```python
from build123d import *

# Parameters (mm, degrees)
BOSS_EXTRUDE1_DEPTH = 80
FILLET1_R           = 1
SKETCH4_R           = 2.05
BOSS_EXTRUDE2_DEPTH = 3.5
BOSS_EXTRUDE3_START = -15
BOSS_EXTRUDE3_DEPTH = 15
SKETCH6_R           = 3.25
CUT_EXTRUDE1_DEPTH  = 44.5
SKETCH8_R           = 1.65
CUT_EXTRUDE2_DEPTH  = 179.465826414


with BuildPart() as part:
    # Sketch1 → Boss-Extrude1 (new body)
    with BuildSketch(Plane.XY):
        with BuildLine():
            Line((-141.65, 83.343364131), (-141.65, 117.256635869))
            Line((-141.65, 117.256635869), (-141.65, 119.95))
            ThreePointArc((-141.65, 119.95), (-141.064213562, 121.364213562), (-139.65, 121.95))
            Line((-139.65, 121.95), (-136.956635869, 121.95))
            Line((-136.956635869, 121.95), (-103.043364131, 121.95))
            Line((-103.043364131, 121.95), (-100.35, 121.95))
            ThreePointArc((-100.35, 121.95), (-98.935786438, 121.364213562), (-98.35, 119.95))
            Line((-98.35, 119.95), (-98.35, 117.256635869))
            Line((-98.35, 117.256635869), (-98.35, 83.343364131))
            Line((-98.35, 83.343364131), (-98.35, 80.65))
            ThreePointArc((-98.35, 80.65), (-98.935786438, 79.235786438), (-100.35, 78.65))
            Line((-100.35, 78.65), (-103.043364131, 78.65))
            Line((-103.043364131, 78.65), (-107.615836726, 78.65))
            ThreePointArc((-107.615836726, 78.65), (-95.926385052, 72.619515209), (-86.80143213, 63.146117643))
            ThreePointArc((-86.80143213, 63.146117643), (-92.047233442, 73.949028976), (-93.85, 85.822164931))
            Line((-93.85, 85.822164931), (-93.85, 121.45))
            ThreePointArc((-93.85, 121.45), (-95.314466094, 124.985533906), (-98.85, 126.45))
            Line((-98.85, 126.45), (-141.15, 126.45))
            ThreePointArc((-141.15, 126.45), (-144.685533906, 124.985533906), (-146.15, 121.45))
            Line((-146.15, 121.45), (-146.15, 85.822164931))
            ThreePointArc((-146.15, 85.822164931), (-147.952766558, 73.949028976), (-153.19856787, 63.146117643))
            ThreePointArc((-153.19856787, 63.146117643), (-144.073614948, 72.619515209), (-132.384163274, 78.65))
            Line((-132.384163274, 78.65), (-136.956635869, 78.65))
            Line((-136.956635869, 78.65), (-139.65, 78.65))
            ThreePointArc((-139.65, 78.65), (-141.064213562, 79.235786438), (-141.65, 80.65))
            Line((-141.65, 80.65), (-141.65, 83.343364131))
        make_face()
    extrude(amount=BOSS_EXTRUDE1_DEPTH)

    # Fillet1
    fillet1_edges = [part.edges().sort_by_distance(p)[0] for p in [
        (-107.615836726, 78.65, 40),
        (-132.384163274, 78.65, 40),
    ]]
    fillet(fillet1_edges, radius=FILLET1_R)

    # Sketch4 → Boss-Extrude2 (add)
    with BuildSketch(Plane(origin=(0, 0, 0), x_dir=(-1, 0, 0), z_dir=(0, 0, -1))):
        with Locations(Location((143, 77.3, 0), (0, 0, 180))):
            Circle(SKETCH4_R)
        with Locations(Location((97, 77.3, 0), (0, 0, 180))):
            Circle(SKETCH4_R)
    extrude(amount=BOSS_EXTRUDE2_DEPTH)

    # Sketch5 → Boss-Extrude3 (add)
    with BuildSketch(Plane.XY.offset(80).offset(BOSS_EXTRUDE3_START)):
        with BuildLine():
            Line((-93.85, 85.822164931), (-93.85, 121.45))
            ThreePointArc((-93.85, 121.45), (-95.314466094, 124.985533906), (-98.85, 126.45))
            Line((-98.85, 126.45), (-141.15, 126.45))
            ThreePointArc((-141.15, 126.45), (-144.685533906, 124.985533906), (-146.15, 121.45))
            Line((-146.15, 121.45), (-146.15, 85.822164931))
            ThreePointArc((-146.15, 85.822164931), (-147.952766558, 73.949028976), (-153.19856787, 63.146117643))
            ThreePointArc((-153.19856787, 63.146117643), (-143.664305463, 72.920402311), (-131.413478874, 78.95))
            Line((-131.413478874, 78.95), (-108.586521126, 78.95))
            ThreePointArc((-108.586521126, 78.95), (-96.335694537, 72.920402311), (-86.80143213, 63.146117643))
            ThreePointArc((-86.80143213, 63.146117643), (-92.047233442, 73.949028976), (-93.85, 85.822164931))
        make_face()
    extrude(amount=BOSS_EXTRUDE3_DEPTH)

    # Sketch6 → Cut-Extrude1 (cut)
    with BuildSketch(Plane(origin=(0, 126.45, 0), x_dir=(1, 0, 0), z_dir=(0, 1, 0))):
        with Locations(Location((-120, -75, 0), (0, 0, 270))):
            Circle(SKETCH6_R)
    extrude(amount=-CUT_EXTRUDE1_DEPTH, mode=Mode.SUBTRACT)

    # Sketch8 → Cut-Extrude2 (cut, through all)
    with BuildSketch(Plane(origin=(0, 81.95, 0), x_dir=(1, 0, 0), z_dir=(0, 1, 0))):
        with Locations(Location((-120, -75, 0), (0, 0, 270))):
            Circle(SKETCH8_R)
    extrude(amount=-CUT_EXTRUDE2_DEPTH, mode=Mode.SUBTRACT)


solid = part.part
```
Input: part model. Units: mm. Frame: model coordinates. A direction names the side the tool comes from. Give positions to 0.01 mm unless a question says otherwise; leave off trailing zeros. Loops run counter-clockwise (first coordinate to the right, second up) from the corner with the lowest first, then second, coordinate; pieces in that order, holes last.
1) Section query C-C on z = 70. Return the cut outline in (x, y), and give its area (3 significant figures).
A:
outline: (-153.2, 63.15) arc R40.3 cw to (-131.41, 78.95) - (-108.59, 78.95) arc R40.3 cw to (-86.8, 63.15) arc R40 cw to (-93.85, 85.82) - (-93.85, 121.45) arc R5 ccw to (-98.85, 126.45) - (-141.15, 126.45) arc R5 ccw to (-146.15, 121.45) - (-146.15, 85.82) arc R40 cw to start
area: 2,610 mm2
2) Reachability of faces 5 (the flat face through (-141.65, 100, 32)), 6 (the flat face through (-146.15, 104, 39)), 7 (the flat face through (-120, 78.95, 72)) from +Z, -Z, +X, -X, +Y, -Y: full face, straight path, thin tool, end or side. Return the list, or none.
A:
face 5: -Z
face 6: +Z, -Z, -X, +Y
face 7: +Z, -Z, -Y
3) Section query A-A on y = 116. Return the cut outline in (x, z), and give its area (3 significant figures).
A:
outline: (-146.15, 0) - (-141.65, 0) - (-141.65, 65) - (-98.35, 65) - (-98.35, 0) - (-93.85, 0) - (-93.85, 80) - (-146.15, 80) - close; hole circle Ø6.5 at (-120, 75)
area: 1,340 mm2
4) Section query B-B on x = -120. Return the cut outline in (y, z).
A:
outline: (78.95, 65) - (121.95, 65) - (121.95, 0) - (126.45, 0) - (126.45, 71.75) - (81.95, 71.75) - (81.95, 73.35) - (78.95, 73.35) - close; (78.95, 76.65) - (81.95, 76.65) - (81.95, 78.25) - (126.45, 78.25) - (126.45, 80) - (78.95, 80) - close
5) Section query D-D on z = 4.5. Return the cut outline in (x, y).
A:
outline: (-153.2, 63.15) arc R40.3 cw to (-137.2, 76.75) arc R1 ccw to (-137.63, 78.65) - (-139.65, 78.65) arc R2 cw to (-141.65, 80.65) - (-141.65, 119.95) arc R2 cw to (-139.65, 121.95) - (-100.35, 121.95) arc R2 cw to (-98.35, 119.95) - (-98.35, 80.65) arc R2 cw to (-100.35, 78.65) - (-102.37, 78.65) arc R1 ccw to (-102.8, 76.75) arc R40.3 cw to (-86.8, 63.15) arc R40 cw to (-93.85, 85.82) - (-93.85, 121.45) arc R5 ccw to (-98.85, 126.45) - (-141.15, 126.45) arc R5 ccw to (-146.15, 121.45) - (-146.15, 85.82) arc R40 cw to start
6) Contact query for flat-ended pins moving along their axis: pin 1 (2 mm diameter, centred on x = -109, y = 101, fed in from -Z); pin 2 (5 mm diameter, centred on x = -99.5, y = 119, fed in from -Z); pin 3 (8 mm diameter, centred on x = -113.5, z = 19.5, fed in from -Y). Output: stop coordinate, or through.
A:
pin 1: stops at z = 65
pin 2: stops at z = 0
pin 3: stops at y = 121.95
7) Line query: L1, parallel to Z at x = -120, y = 79; L2, parallel to X at y = 100, z = 75; L3, parallel to X at y = 98.5, z = 54. Output: solid intervals per line, ascending.
A:
L1: z = 65 to 73.35, 76.65 to 80
L2: x = -146.15 to -123.25, -116.75 to -93.85
L3: x = -146.15 to -141.65, -98.35 to -93.85
8) Mould query, pull axis Y, two halves, no side actions, for faces 1 (the cylindrical face through (-141.05, 79.22, 32.04)), 2 (the cylindrical face through (-98.5, 75.9, -1.7)), 3 (the flat face through (-143, 77, -3.5)), 4 (the cylindrical face through (-147.903, 74.11, 39.44)). Classes: released by +Y, released by -Y, zero draft, split by the parting line, or undercut.
A:
face 1: undercut
face 2: split by the parting line
face 3: zero draft
face 4: released by +Y
